from build123d import *

# Parameters (mm, degrees)
SKETCH1_W           = 740
SKETCH1_H           = 145
BOSS_EXTRUDE1_DEPTH = 34
SKETCH2_R           = 3
CUT_EXTRUDE1_DEPTH  = 379.566044436
CUT_EXTRUDE2_DEPTH  = 379.566044436
CUT_EXTRUDE3_DEPTH  = 9
CUT_EXTRUDE4_DEPTH  = 9


with BuildPart() as part:
    # Sketch1 → Boss-Extrude1 (new body)
    with BuildSketch(Plane.XY):
        Rectangle(SKETCH1_W, SKETCH1_H)
    extrude(amount=BOSS_EXTRUDE1_DEPTH)

    # Sketch2 → Cut-Extrude1 (cut, through all)
    with BuildSketch(Plane.XY.offset(34)):
        with Locations((-300, 0)):
            Circle(SKETCH2_R)
    cut_extrude1 = extrude(amount=-CUT_EXTRUDE1_DEPTH, mode=Mode.SUBTRACT)

    # Mirror1: Cut-Extrude1 across plane
    add(cut_extrude1.mirror(Plane(origin=(0, 0, 0), x_dir=(0, 0, 1), z_dir=(1, 0, 0))), mode=Mode.SUBTRACT)

    # Sketch3 → Cut-Extrude2 (cut, through all)
    with BuildSketch(Plane(origin=(0, 0, 0), x_dir=(-1, 0, 0), z_dir=(0, 0, -1))):
        Polygon((-370, 1.769559051), (-300.776712208, -72.5), (-300.776712208, -90.031965517), (-434.728473362, -90.031965517), (-434.728473362, 1.769559051), align=None)
        Polygon((300.776712208, -72.5), (370, 1.769559051), (452.615528046, -36.803788203), (398.593275425, -163.670382496), align=None)
    extrude(amount=-CUT_EXTRUDE2_DEPTH, mode=Mode.SUBTRACT)

    # Sketch4 → Cut-Extrude3 (cut)
    with BuildSketch(Plane.XY.offset(34)):
        Polygon((-485.714618039, 114.044241674), (-337.944791384, 114.044241674), (-115.198220107, -124.940212205), (-485.714618039, -111.910111467), align=None)
    extrude(amount=-CUT_EXTRUDE3_DEPTH, mode=Mode.SUBTRACT)

    # Sketch5 → Cut-Extrude4 (cut)
    with BuildSketch(Plane(origin=(0, 0, 0), x_dir=(-1, 0, 0), z_dir=(0, 0, -1))):
        Polygon((-568.705938923, 127.353116935), (-361.833214072, 139.674093651), (-111.696100657, -128.697630779), (-536.326991512, -147.10621474), align=None)
    extrude(amount=-CUT_EXTRUDE4_DEPTH, mode=Mode.SUBTRACT)


solid = part.part
Check sheet for the modelled part. Datum: model origin and axes. Units: mm. A direction names the side the tool comes from. Give positions to 0.01 mm unless a question says otherwise; leave off trailing zeros. Order: outer loops, then holes, each group sorted by start corner. A loop starts at its lowest first (then second) coordinate and runs counter-clockwise, first axis right, second up. Notation, with made-up numbers: (26, -15.75) - (38, -15.75) arc R22 ccw to (38, -6.75) - close; hole circle Ø10 at (26.25, -12). An arc over 180 degrees is marked (long way). Answer as CSV lines item,"result".
1. Section check B-B (x = -188). Record the boundary of the cut face in (y, z), then the cut area to 3 significant figures.
Result sheet:
outline,"(-72.5, 0) - (72.5, 0) - (72.5, 34) - (-46.83, 34) - (-46.83, 25) - (-72.5, 25) - close"
area,"4,700 mm²"
2. Tool access check on faces 1 (the face through (31, 1, 34)), 2 (the face through (-232.6, 1.02, 29.56)), 3 (the face through (232.595, 1.015, 4.437)). Record the directions out of +Z, -Z, +X, -X, +Y, -Y that give a thin tool (end or side, any length) a straight path to the whole face; none if there is none.
Result sheet:
face 1,"+Z, +X, -X, +Y, -Y"
face 2,"+Z, -X, -Y"
face 3,"-Z, +X, -Y"
3. Section check A-A (y = -33.5). Record the boundary of the cut face in (x, z), then the cut area to 3 significant figures.
Result sheet:
outline,"(-337.13, 0) - (200.43, 0) - (200.43, 9) - (337.13, 9) - (337.13, 34) - (-200.43, 34) - (-200.43, 25) - (-337.13, 25) - close"
area,"20,500 mm²"
4. Scan lines: probe 1 along Y at (x, z) = (300, 23); probe 2 along Z at (x, y) = (292.5, 34); probe 3 along X at (y, z) = (0, 27). Record each from-to range of solid material in increasing order. Write a range as from..to.
Result sheet:
probe 1,"-72.5..-3, 3..72.5"
probe 2,"9..34"
probe 3,"-231.65..297, 303..368.35"
